The model under review builds one solid part; all positions refer to its coordinate system, in mm. A direction names the side the tool comes from. Round coordinates to 2 decimals unless told otherwise and drop trailing zeros. Loops run counter-clockwise (first coordinate to the right, second up) from the corner with the lowest first, then second, coordinate; pieces in that order, holes last. Notation, with made-up numbers: M 26,7 L 58,7 A29 ccw 58,31 Z; hole C 74.5,69 d10. An arc over 180 degrees is marked long. Return JSON: item names as keys, results as strings. Group by question number.
Q1. Consider section A-A (y = -95.5). State the section outline as (x, z) points.
Q2. To check wall thickness, follow line 1 along Y through (x, z) = (-63, 8.25); line 2 along Z through (x, y) = (5.5, 100.5); line 3 along Y through (x, z) = (8, 2.25). State the ranges of each line that lie inside material, in increasing order.
Q3. Consider section C-C (x = -18.5). State the section outline as (y, z) points.
Q4. For faces 1 (the face through (-48, -20.464, 0)), 2 (the face through (-49, 28, -9.997)), 3 (the face through (-67.885, 28.037, -0.264)), 4 (the face through (12.52, -104.21, -6.04)), 5 (the face through (-10, 9, 9.906)), list the 3-axis set-ups (+Z, -Z, +X, -X, +Y, -Y) from which the entire face can be reached by the end or side of a thin tool; tool diameter is ignored.
Q5. Consider section B-B (x = 8). Count the separate pieces of the cut face and the enclosed holes in it, and give its area (3 significant figures).
Q6. Draft analysis for pull direction Z (two halves, no side actions). For faces 6 (the face through (-67.687, -28.577, 0.46)), 7 (the face through (13, -1, -13.887)), 8 (the face through (-34, -36.466, 0)), 9 (the face through (12.52, -94.3, -5.28)), state which applies: pulls with the +Z half, pulls with the -Z half, needs draft (parallel to the pull), parting line crosses it, or undercut.
Q7. Clearance check with flat-ended pins moving along their axes: pin 1 Ø9.5 at (x, y) = (-45, -28) entering from +Z; pin 2 Ø6 at (x, z) = (-50.5, -0.5) entering from +Y; pin 3 Ø8 at (x, z) = (4.5, -10.5) entering from -Y. State where each tip first meets the part, or that it passes through.
Q8. Consider section D-D (y = 33.5). State the section outline as (x, z) points, and give its area (3 significant figures).
from build123d import *

# Parameters (mm, degrees)
F1_DEPTH = 25.4
F3_DEPTH = 9.906
F4_R     = 5.4054687582
F5_DEPTH = 17.018
F7_DEPTH = 16.002


# Not quite as in the source:
# - ends of sketch curves that miss each other by under 0.0002 mm in the source are joined


with BuildPart() as f1:
    # F0 (on Right) → F1 (new body)
    with BuildSketch(Plane.YZ):
        with BuildLine():
            Line((-99.6930599213, 7.5515317731), (-99.6930599213, 13.8873864871))
            ThreePointArc((-99.6930599213, 13.8873864871), (-113.5804464084, 0), (-99.6930599213, -13.8873864871))
            Line((-99.6930599213, -13.8873864871), (-99.6930599213, -7.5509602816))
            ThreePointArc((-99.6930599213, -7.5509602816), (-104.2631477896, -6.0002098207), (-106.9606792933, -1.9984784576))
            ThreePointArc((-106.9606792933, -1.9984784576), (-107.2304460851, -0.0041593028), (-106.9628804792, 1.9904563644))
            ThreePointArc((-106.9628804792, 1.9904563644), (-104.2749842635, 5.9848237142), (-99.7176355394, 7.5373431398))
            ThreePointArc((-99.7176355394, 7.5373431398), (-99.7053477533, 7.5373772953), (-99.6930599213, 7.5373873115))
            Line((-99.6930599213, 7.5373873115), (-99.6930599213, 7.5515317731))
        make_face()
        with BuildLine():
            Line((99.6930599213, 13.8873864871), (-99.6930599213, 13.8873864871))
            Line((-99.6930599213, 13.8873864871), (-99.6930599213, 7.5515317731))
            ThreePointArc((-99.6930599213, 7.5515317731), (-94.3533205962, 5.3397393251), (-92.1415281482, 0))
            ThreePointArc((-92.1415281482, 0), (-94.3541776231, -5.33475565), (-99.6930599995, -7.5374291426))
            Line((-99.6930599995, -7.5374291426), (-99.6930599213, -7.5509602816))
            Line((-99.6930599213, -7.5509602816), (-99.6930599213, -13.8873864871))
            Line((-99.6930599213, -13.8873864871), (99.6930599213, -13.8873864871))
            Line((99.6930599213, -13.8873864871), (99.6930599213, -7.671022612))
            ThreePointArc((99.6930599213, -7.671022612), (94.2688278137, -5.4242321076), (92.0220373093, 0))
            ThreePointArc((92.0220373093, 0), (92.1497116605, 1.39373058), (92.5284847617, 2.7410674375))
            ThreePointArc((92.5284847617, 2.7410674375), (95.3446235575, 6.3194690523), (99.6930599213, 7.671022612))
            Line((99.6930599213, 7.671022612), (99.6930599213, 13.8873864871))
        make_face()
        with BuildLine():
            ThreePointArc((99.6930599213, -13.8873864871), (113.5804464084, 0), (99.6930599213, 13.8873864871))
            Line((99.6930599213, 13.8873864871), (99.6930599213, 7.671022612))
            ThreePointArc((99.6930599213, 7.671022612), (107.3640825332, 0), (99.6930599213, -7.671022612))
            Line((99.6930599213, -7.671022612), (99.6930599213, -13.8873864871))
        make_face()
    extrude(amount=F1_DEPTH)

    # F2 (on Top) → F3 (join, symmetric)
    with BuildSketch(Plane.XY):
        with BuildLine():
            Line((0, 0), (0, 36.4271812141))
            Line((0, 36.4271812141), (-39.9832986295, 36.4271812141))
            Line((-39.9832986295, 36.4271812141), (-39.9832986295, 19.475013286))
            ThreePointArc((-39.9832986295, 19.475013286), (-13.9090954175, -0.413186714), (-39.9832986295, -20.301386714))
            Line((-39.9832986295, -20.301386714), (-39.9832986295, -36.4658497274))
            Line((-39.9832986295, -36.4658497274), (0, -36.4658497274))
            Line((0, -36.4658497274), (0, -36.4271812141))
            Line((0, -36.4271812141), (0, 0))
        make_face()
    extrude(amount=F3_DEPTH, both=True)

    # F4 (on face) → F5 (join)
    with BuildSketch(Plane(origin=(0, 36.4271812141, 0), x_dir=(-1, 0, 0), z_dir=(0, 1, 0))):
        with BuildLine():
            Line((57.9356960952, 9.906), (39.9832986295, 9.906))
            Line((39.9832986295, 9.906), (39.9832986295, -9.906))
            Line((39.9832986295, -9.906), (39.9832986295, -9.9966842681))
            Line((39.9832986295, -9.9966842681), (57.9356960952, -9.9966842681))
            ThreePointArc((57.9356960952, -9.9966842681), (67.8870382293, -0.0453421341), (57.9356960952, 9.906))
        make_face()
        with Locations((57.9356960952, -0.0453421341)):
            Circle(F4_R, mode=Mode.SUBTRACT)
    extrude(amount=-F5_DEPTH)

    # F6 (on face) → F7 (join)
    with BuildSketch(Plane.XZ.offset(36.4658497274)):
        with BuildLine():
            Line((-52.1078817546, -9.906), (-39.9832986295, -9.906))
            Line((-39.9832986295, -9.906), (-39.9832986295, 9.906))
            Line((-39.9832986295, 9.906), (-39.9832986295, 10.2091357112))
            Line((-39.9832986295, 10.2091357112), (-52.1078817546, 10.2091357112))
            Line((-52.1078817546, 10.2091357112), (-52.1078817546, 5.8468863204))
            ThreePointArc((-52.1078817546, 5.8468863204), (-50.0877827712, 3.3118599928), (-49.366872241, 0.1515678556))
            ThreePointArc((-49.366872241, 0.1515678556), (-50.0877827712, -3.0087242816), (-52.1078817546, -5.5437506092))
            Line((-52.1078817546, -5.5437506092), (-52.1078817546, -9.906))
        make_face()
        with BuildLine():
            ThreePointArc((-52.1078817546, 10.2091357112), (-67.6917094663, 0.1515678556), (-52.1078817546, -9.906))
            Line((-52.1078817546, -9.906), (-52.1078817546, -5.5437506092))
            ThreePointArc((-52.1078817546, -5.5437506092), (-63.9417160607, 0.1515678556), (-52.1078817546, 5.8468863204))
            Line((-52.1078817546, 5.8468863204), (-52.1078817546, 10.2091357112))
        make_face()
    extrude(amount=-F7_DEPTH)


solid = f1.part
Values:
{
 "1": {"outline": "M 0,-13.89 L 25.4,-13.89 L 25.4,-6.27 L 0,-6.27 Z; M 0,6.28 L 25.4,6.28 L 25.4,13.89 L 0,13.89 Z"},
 "2": {"line 1": "y = -36.47 to -20.46, 19.41 to 36.43", "line 2": "z = -13.86 to -7.63, 7.63 to 13.86", "line 3": "y = -113.4 to -106.89, -92.48 to 92.36, 107.03 to 113.4"},
 "3": {"outline": "M -36.47,-9.91 L -13.39,-9.91 L -13.39,9.91 L -36.47,9.91 Z; M 12.56,-9.91 L 36.43,-9.91 L 36.43,9.91 L 12.56,9.91 Z"},
 "4": {"face 1": "+Z, -Z, -X", "face 2": "-Z, -X, +Y", "face 3": "-X, +Y", "face 4": "+X, -X", "face 5": "+Z, +Y"},
 "5": {"separate pieces": "1", "enclosed holes": "2", "area": "5,780 mm2"},
 "6": {"face 6": "parting line crosses it", "face 7": "pulls with the -Z half", "face 8": "needs draft", "face 9": "undercut"},
 "7": {"pin 1": "stops at z = 10.21", "pin 2": "stops at y = 36.43", "pin 3": "stops at y = -111.97"},
 "8": {"outline": "M -57.94,-10 L -39.98,-10 L -39.98,-9.91 L 0,-9.91 L 0,-13.89 L 25.4,-13.89 L 25.4,13.89 L 0,13.89 L 0,9.91 L -57.94,9.91 A9.95 ccw Z; hole C -57.94,-0.05 d10.81", "area": "1,920 mm2"}
}
